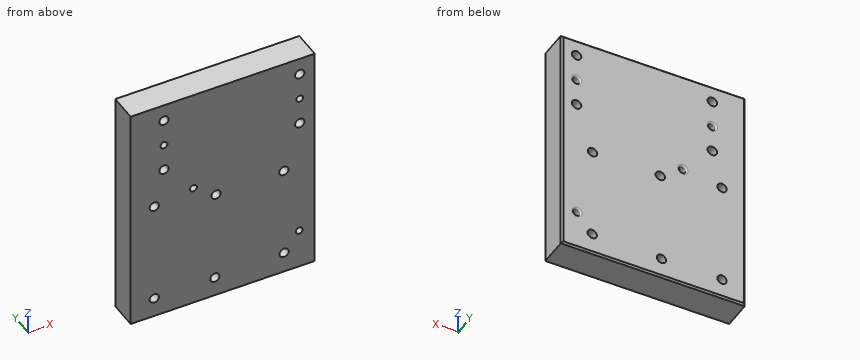
```python
from build123d import *

# Parameters (mm, degrees)
SKETCH1_W           = 160
SKETCH1_H           = 203
SKETCH1_R           = 4.05
SKETCH1_R_2         = 4.1
SKETCH1_R_3         = 3
BOSS_EXTRUDE1_DEPTH = 26
FILLET1_R           = 1.5
CHAMFER1_SIZE       = 1.5


with BuildPart() as part:
    # Sketch1 → Boss-Extrude1 (new body)
    with BuildSketch(Plane(origin=(0, 0, 0), x_dir=(1, 0, 0), z_dir=(0, 1, 0))):
        with Locations((80.434245342, 28.5)):
            Rectangle(SKETCH1_W, SKETCH1_H)
        with Locations(Location((73.68, 112.78, 0), (0, 0, 90))):
            Circle(SKETCH1_R, mode=Mode.SUBTRACT)
        with Locations(Location((133.87, 111.67, 0), (0, 0, 90))):
            Circle(SKETCH1_R, mode=Mode.SUBTRACT)
        with Locations(Location((133.61, 31.48, 0), (0, 0, 90))):
            Circle(SKETCH1_R, mode=Mode.SUBTRACT)
        with Locations(Location((74.69, 31.92, 0), (0, 0, 90))):
            Circle(SKETCH1_R, mode=Mode.SUBTRACT)
        with Locations(Location((29.434245342, -10, 0), (0, 0, 90))):
            Circle(SKETCH1_R_2, mode=Mode.SUBTRACT)
        with Locations(Location((29.434245342, -58, 0), (0, 0, 90))):
            Circle(SKETCH1_R_2, mode=Mode.SUBTRACT)
        with Locations(Location((21, 112.78, 0), (0, 0, 90))):
            Circle(SKETCH1_R, mode=Mode.SUBTRACT)
        with Locations(Location((147.434245342, -58, 0), (0, 0, 90))):
            Circle(SKETCH1_R_2, mode=Mode.SUBTRACT)
        with Locations(Location((147.434245342, -10, 0), (0, 0, 90))):
            Circle(SKETCH1_R_2, mode=Mode.SUBTRACT)
        with Locations(Location((21, 23, 0), (0, 0, 90))):
            Circle(SKETCH1_R, mode=Mode.SUBTRACT)
        with Locations(Location((29.434245342, -34, 0), (0, 0, 90))):
            Circle(SKETCH1_R_3, mode=Mode.SUBTRACT)
        with Locations(Location((147.434245342, -34, 0), (0, 0, 90))):
            Circle(SKETCH1_R_3, mode=Mode.SUBTRACT)
        with Locations(Location((147, 95, 0), (0, 0, 90))):
            Circle(SKETCH1_R_3, mode=Mode.SUBTRACT)
        with Locations(Location((55, 18, 0), (0, 0, 90))):
            Circle(SKETCH1_R_3, mode=Mode.SUBTRACT)
    extrude(amount=BOSS_EXTRUDE1_DEPTH)

    # Fillet1
    fillet1_edges = [part.edges().sort_by_distance(p)[0] for p in [
        (29.434245342, 26, 37),
        (147.434245342, 26, 37),
        (147, 26, -92),
        (55, 26, -15),
    ]]
    fillet(fillet1_edges, radius=FILLET1_R)

    # Chamfer1
    chamfer1_edges = [part.edges().sort_by_distance(p)[0] for p in [
        (0.434245342, 26, -28.5),
        (80.434245342, 26, 73),
        (160.434245342, 26, -28.5),
        (80.434245342, 26, -130),
    ]]
    chamfer(chamfer1_edges, length=CHAMFER1_SIZE)


solid = part.part
```
Source: CAD feature listing. Evaluate the final solid. Frame: model axes, mm. Round coordinates to 2 decimals unless told otherwise and drop trailing zeros. Write each loop counter-clockwise with the first axis right and the second up, starting at its lowest first coordinate (ties: lowest second). Pieces come first, ordered by that corner, then holes. Notation, with made-up numbers: M 76,-25.75 L 135,-25.75 A28 ccw 135,12.25 Z; hole C 82.5,18.25 d10. An arc over 180 degrees is marked long. Answer as a JSON object with one key per item and string values. Group by question number.
(1) Section query A-A on z = 10. Output: boundary loops of the cut face in (x, y), then the cut area to 3 significant figures.
(2) Ray query, line 1 (X direction, y = 12.25, z = -31.92); line 2 (X direction, y = 9, z = -31.48); line 3 (Z direction, x = 21, y = 19.25). Return the intervals inside material, ascending. Write a range as [from, to].
(3) First-contact query: pin 1 (5 mm diameter, centred on x = 55, z = -18, fed in from -Y). Flat tip, straight axial feed; report the tip coordinate or a pass-through.
(4) Section query C-C on z = -111.67. Output: boundary loops of the cut face in (x, y).
(5) Section query B-B on y = 22. State how many separate pieces and enclosed holes the cut face has, then the cut area to 3 significant figures.
Computed values:
{
 "1": {"outline": "M 0.43,0 L 25.33,0 L 25.33,26 L 1.93,26 L 0.43,24.5 Z; M 33.53,0 L 143.33,0 L 143.33,26 L 33.53,26 Z; M 151.53,0 L 160.43,0 L 160.43,24.5 L 158.93,26 L 151.53,26 Z", "area": "3,730 mm^2"},
 "2": {"line 1": "[0.43, 70.64], [78.74, 129.58], [137.64, 160.43]", "line 2": "[0.43, 70.66], [78.72, 129.56], [137.66, 160.43]", "line 3": "[-130, -116.83], [-108.73, -27.05], [-18.95, 73]"},
 "3": {"pin 1": "through"},
 "4": {"outline": "M 0.43,0 L 17.11,0 L 17.11,26 L 1.93,26 L 0.43,24.5 Z; M 24.89,0 L 69.79,0 L 69.79,26 L 24.89,26 Z; M 77.57,0 L 129.82,0 L 129.82,26 L 77.57,26 Z; M 137.92,0 L 160.43,0 L 160.43,24.5 L 158.93,26 L 137.92,26 Z"},
 "5": {"separate pieces": "1", "enclosed holes": "14", "area": "31,800 mm^2"}
}
